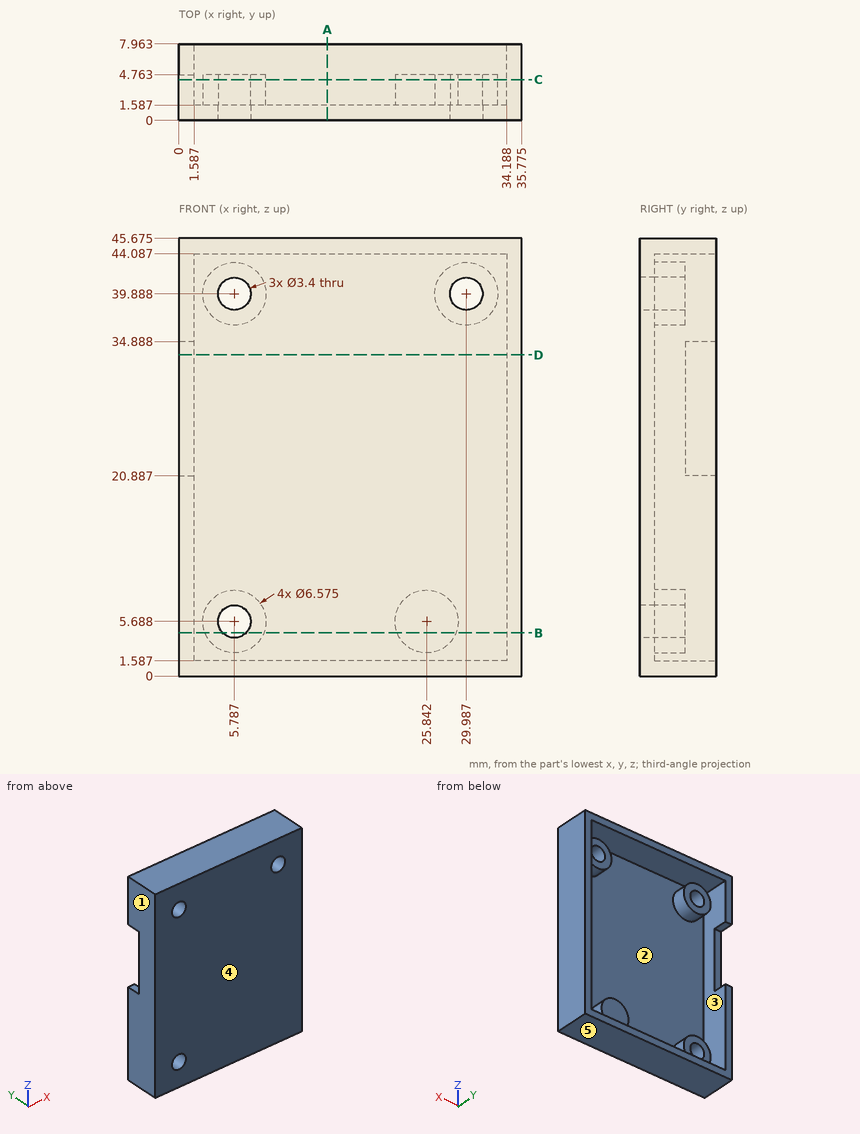
Design review of the part shown in the three views and the two pictorial views. Dimensions are in mm from the part's minimum x, y and z. A direction names the side the tool comes from. Give positions to 0.01 mm unless a question says otherwise; leave off trailing zeros. Loops run counter-clockwise (first coordinate to the right, second up) from the corner with the lowest first, then second, coordinate; pieces in that order, holes last. Notation, with made-up numbers: (-2.75, 14.5) - (38.25, 14.5) arc R20 ccw to (38.25, 53.5) - close; hole circle Ø1 at (25, 39). An arc over 180 degrees is marked (long way). Write item = value, one per line.
1) Draft analysis for pull direction Z (two halves, no side actions). For the marked faces 3, 4 and 5, state which applies: +Z half, -Z half, draft (parallel to the pull), parting line (faces both ways), or undercut.
Result sheet:
face_3 = undercut
face_4 = draft
face_5 = -Z half
2) Take a section at D-D on z = 33.5. State the section outline as (x, y) points (1 decimal).
Result sheet:
outline = (0, 0) - (35.8, 0) - (35.8, 8) - (34.2, 8) - (34.2, 1.6) - (1.6, 1.6) - (1.6, 4.8) - (0, 4.8) - close
3) Take a section at B-B on z = 4.5. State the section outline as (x, y) points (1 decimal), and give its area (3 significant figures).
Result sheet:
outline = (0, 0) - (4.6, 0) - (4.6, 4.8) - (2.7, 4.8) - (2.7, 1.6) - (1.6, 1.6) - (1.6, 8) - (0, 8) - close; (7, 0) - (35.8, 0) - (35.8, 8) - (34.2, 8) - (34.2, 1.6) - (28.9, 1.6) - (28.9, 4.8) - (22.8, 4.8) - (22.8, 1.6) - (8.9, 1.6) - (8.9, 4.8) - (7, 4.8) - close
area = 104 mm2
4) Take a section at C-C on y = 4.25. Count the separate pieces of the cut face and the enclosed holes in it.
Result sheet:
separate_pieces = 5
enclosed_holes = 4
5) Clearance check with flat-ended pins moving along their axes: pin 1 Ø0.5 at (x, y) = (0.5, 7) entering from -Z; pin 2 Ø1.7 at (x, z) = (1, 29) entering from +Y; pin 3 Ø2 at (y, z) = (6.5, 28) entering from -X; pin 4 Ø1.5 at (x, z) = (22, 36.5) entering from +Y. State where each tip first meets the part, or that it passes through.
Result sheet:
pin_1 = 0
pin_2 = 4.76
pin_3 = 34.19
pin_4 = 1.59
6) Take a section at A-A on x = 15.5. State the section outline as (y, z) points (1 decimal).
Result sheet:
outline = (0, 0) - (8, 0) - (8, 1.6) - (1.6, 1.6) - (1.6, 44.1) - (8, 44.1) - (8, 45.7) - (0, 45.7) - close
7) To check wall thickness, follow line 1 (X direction, y = 7.25, z = 3.5) (1 decimal); line 2 (Z direction, x = 17, y = 1.75) (1 decimal); line 3 (Z direction, x = 28, y = 3.5) (1 decimal). State the ranges of each line that lie inside material, in increasing order.
Result sheet:
line_1 = 0 to 1.6, 34.2 to 35.8
line_2 = 0 to 1.6, 44.1 to 45.7
line_3 = 0 to 1.6, 3.2 to 8.2, 37.3 to 42.5, 44.1 to 45.7
8) Tool access review of the marked faces 1 and 2: name each direction out of +Z, -Z, +X, -X, +Y, -Y from which nothing blocks a thin tool from reaching the whole face with its end or side.
Result sheet:
face_1 = +Z, -Z, -X, +Y, -Y
face_2 = +Y
